```python
from build123d import *

# Parameters (mm, degrees)
SKETCH_1_R                = 65
EXTRUDE_1_DEPTH           = 15
SKETCH_2_R                = 45
CUT_EXTRUDE_1_DEPTH       = 15
SKETCH_3_R                = 53
CUT_EXTRUDE_2_DEPTH       = 2
HOLE_WIZARD_1_D           = 4.5
HOLE_WIZARD_1_CBORE_D     = 8
HOLE_WIZARD_1_CBORE_DEPTH = 4.6
PATTERN_CIRCULAR_1_COUNT  = 10
HOLE_WIZARD_2_D           = 4.5
HOLE_WIZARD_2_CBORE_D     = 8
HOLE_WIZARD_2_CBORE_DEPTH = 4.6
PATTERN_CIRCULAR_2_COUNT  = 10


with BuildPart() as part:
    # Sketch 1 → Extrude 1 (new body)
    with BuildSketch(Plane.XY):
        Circle(SKETCH_1_R)
    extrude(amount=EXTRUDE_1_DEPTH)

    # Sketch 2 → Cut-Extrude 1 (cut)
    with BuildSketch(Plane(origin=(0, 0, 0), x_dir=(-1, 0, 0), z_dir=(0, 0, -1))):
        Circle(SKETCH_2_R)
    extrude(amount=-CUT_EXTRUDE_1_DEPTH, mode=Mode.SUBTRACT)

    # Sketch 3 → Cut-Extrude 2 (cut)
    with BuildSketch(Plane(origin=(0, 0, 0), x_dir=(-1, 0, 0), z_dir=(0, 0, -1))):
        Circle(SKETCH_3_R)
    extrude(amount=-CUT_EXTRUDE_2_DEPTH, mode=Mode.SUBTRACT)

    # Hole Wizard 1 (through all)
    with Locations(Plane.XY.offset(15)):
        with Locations((0, 50)):
            hole_wizard_1 = CounterBoreHole(HOLE_WIZARD_1_D / 2, HOLE_WIZARD_1_CBORE_D / 2, HOLE_WIZARD_1_CBORE_DEPTH)

    # Pattern Circular 1: Hole Wizard 1 ×10 about axis
    pattern_circular_1_axis = Axis((0, 0, 0), (0, 0, 1))
    for i in range(1, PATTERN_CIRCULAR_1_COUNT):
        add(hole_wizard_1.rotate(pattern_circular_1_axis, i * 360 / PATTERN_CIRCULAR_1_COUNT), mode=Mode.SUBTRACT)

    # Hole Wizard 2 (through all)
    with Locations(Plane(origin=(0, 0, 0), x_dir=(-1, 0, 0), z_dir=(0, 0, -1))):
        with Locations((-18.541019662, 57.063390978)):
            hole_wizard_2 = CounterBoreHole(HOLE_WIZARD_2_D / 2, HOLE_WIZARD_2_CBORE_D / 2, HOLE_WIZARD_2_CBORE_DEPTH)

    # Pattern Circular 2: Hole Wizard 2 ×10 about axis
    pattern_circular_2_axis = Axis((0, 0, 0), (0, 0, 1))
    for i in range(1, PATTERN_CIRCULAR_2_COUNT):
        add(hole_wizard_2.rotate(pattern_circular_2_axis, i * 360 / PATTERN_CIRCULAR_2_COUNT), mode=Mode.SUBTRACT)


solid = part.part
```
Geometry: final body of the model. Coordinates: model frame, mm. A direction names the side the tool comes from. Give positions to 0.01 mm unless a question says otherwise; leave off trailing zeros. Loops run counter-clockwise (first coordinate to the right, second up) from the corner with the lowest first, then second, coordinate; pieces in that order, holes last. Notation, with made-up numbers: (60.5, -25.75) -> (100.5, -25.75) arc R21 cw to (100.5, -5.75) -> close; hole circle Ø8 at (-29, -4.5). An arc over 180 degrees is marked (long way). Use CSV: the item, a comma, the result in double quotes.
(1) Cut plane B-B (y = 0). Output: boundary loops of the cut face in (x, z).
From the geometry:
outline,"(-65, 0) -> (-64, 0) -> (-64, 4.6) -> (-62.25, 4.6) -> (-62.25, 15) -> (-65, 15) -> close; (-57.75, 4.6) -> (-56, 4.6) -> (-56, 0) -> (-53, 0) -> (-53, 2) -> (-45, 2) -> (-45, 15) -> (-57.75, 15) -> close; (45, 2) -> (53, 2) -> (53, 0) -> (56, 0) -> (56, 4.6) -> (57.75, 4.6) -> (57.75, 15) -> (45, 15) -> close; (62.25, 4.6) -> (64, 4.6) -> (64, 0) -> (65, 0) -> (65, 15) -> (62.25, 15) -> close"
(2) Cut plane C-C (y = -50). Output: boundary loops of the cut face in (x, z).
From the geometry:
outline,"(-41.53, 0) -> (-17.58, 0) -> (-17.58, 2) -> (-2.25, 2) -> (-2.25, 10.4) -> (-4, 10.4) -> (-4, 15) -> (-41.53, 15) -> close; (2.25, 2) -> (17.58, 2) -> (17.58, 0) -> (41.53, 0) -> (41.53, 15) -> (4, 15) -> (4, 10.4) -> (2.25, 10.4) -> close"
(3) Access query for faces 1 (the face through (43.607, -16.11, 12.732)), 2 (the face through (-47, 33, 4.6)), 3 (the face through (-50.635, -36.091, 9.873)). Directions: +Z, -Z, +X, -X, +Y, -Y. A direction counts if a zero-diameter tool reaches every point of the face in a straight line with its end or side. Return the directions, or none.
From the geometry:
face 1,"+Z"
face 2,"-Z"
face 3,"+Z, -Z"
(4) Pull-direction query (X, two-part tool) for faces 4 (the face through (62, 19.52, 7.4)), 5 (the face through (57.8, 1.1, 4.6)); classes: released by +X, released by -X, zero draft, split by the parting line, or undercut.
From the geometry:
face 4,"split by the parting line"
face 5,"undercut"
(5) First-contact query: P1, Ø6.5, axis at x = -18.54, y = 57.06, coming from the -Z side; P2, Ø2.5, axis at x = -48.5, y = -16, coming from the +Z side; P3, Ø1.5, axis at x = 25, y = -43, coming from the -Z side. Flat tips, straight axial feed; report the tip coordinate or a pass-through.
From the geometry:
P1,"z = 4.6"
P2,"z = 10.4"
P3,"z = 2"
(6) Ray query, line 1 along Y through (x, z) = (0, 13.1); line 2 along X through (y, z) = (2.5, 1); line 3 along Y through (x, z) = (19, 7). Return the intervals inside material, ascending. Write a range as [from, to].
From the geometry:
line 1,"[-65, -54], [-46, -45], [45, 46], [54, 65]"
line 2,"[-64.95, -63.12], [-56.88, -52.94], [52.94, 56.88], [63.12, 64.95]"
line 3,"[-62.16, -59.27], [-54.86, -40.79], [40.79, 54.86], [59.27, 62.16]"
(7) Cut plane A-A (x = 0). Output: boundary loops of the cut face in (y, z), plus the area to 3 significant figures.
From the geometry:
outline,"(-65, 0) -> (-53, 0) -> (-53, 2) -> (-52.25, 2) -> (-52.25, 10.4) -> (-54, 10.4) -> (-54, 15) -> (-65, 15) -> close; (-47.75, 2) -> (-45, 2) -> (-45, 15) -> (-46, 15) -> (-46, 10.4) -> (-47.75, 10.4) -> close; (45, 2) -> (47.75, 2) -> (47.75, 10.4) -> (46, 10.4) -> (46, 15) -> (45, 15) -> close; (52.25, 2) -> (53, 2) -> (53, 0) -> (65, 0) -> (65, 15) -> (54, 15) -> (54, 10.4) -> (52.25, 10.4) -> close"
area,"419 mm^2"
(8) Cut plane D-D (z = 12.25). Count the separate pieces of the cut face and the enclosed holes in it, plus the area to 3 significant figures.
From the geometry:
separate pieces,"1"
enclosed holes,"21"
area,"6,250 mm^2"
